Study the drawing (mm; zero at the part's minimum x, y, z) and answer. Coordinates: 2 decimals unless noted, no trailing zeros. Order: outer loops, then holes, each group sorted by start corner. A loop starts at its lowest first (then second) coordinate and runs counter-clockwise, first axis right, second up.
1. The part is cut by section C-C, the plane y = 1. Give the vertices of the cut face in (x, z), then the cut area to 3 significant figures.
2. Flat-ended cylindrical pins translate along their axes: pin 1 Ø2 at (x, z) = (9, 9) entering from -Y; pin 2 Ø8 at (y, z) = (7, 7) entering from -X; pin 3 Ø5.5 at (x, z) = (7.5, 6) entering from +Y; pin 4 Ø1 at (x, z) = (3, 10.5) entering from +Y. Find the tip coordinate at first contact, or state that the pin passes through.
3. Find the intervals of material crossed by probe 1 along X at (y, z) = (6.25, 9); probe 2 along Y at (x, z) = (13.5, 2.5), in increasing order.
4. The part is cut by section D-D, the plane z = 11. Give the vertices of the cut face in (x, y).
5. Determine the mould class of the marked faces 1, 2 and 3 for opening direction Z: +Z half, -Z half, draft (parallel to the pull), parting line (faces both ways), or undercut.
6. The part is cut by section B-B, the plane z = 9. Give the vertices of the cut face in (x, y), then the cut area to 4 significant figures.
7. The part is cut by section A-A, the plane x = 9. Give the vertices of the cut face in (y, z).
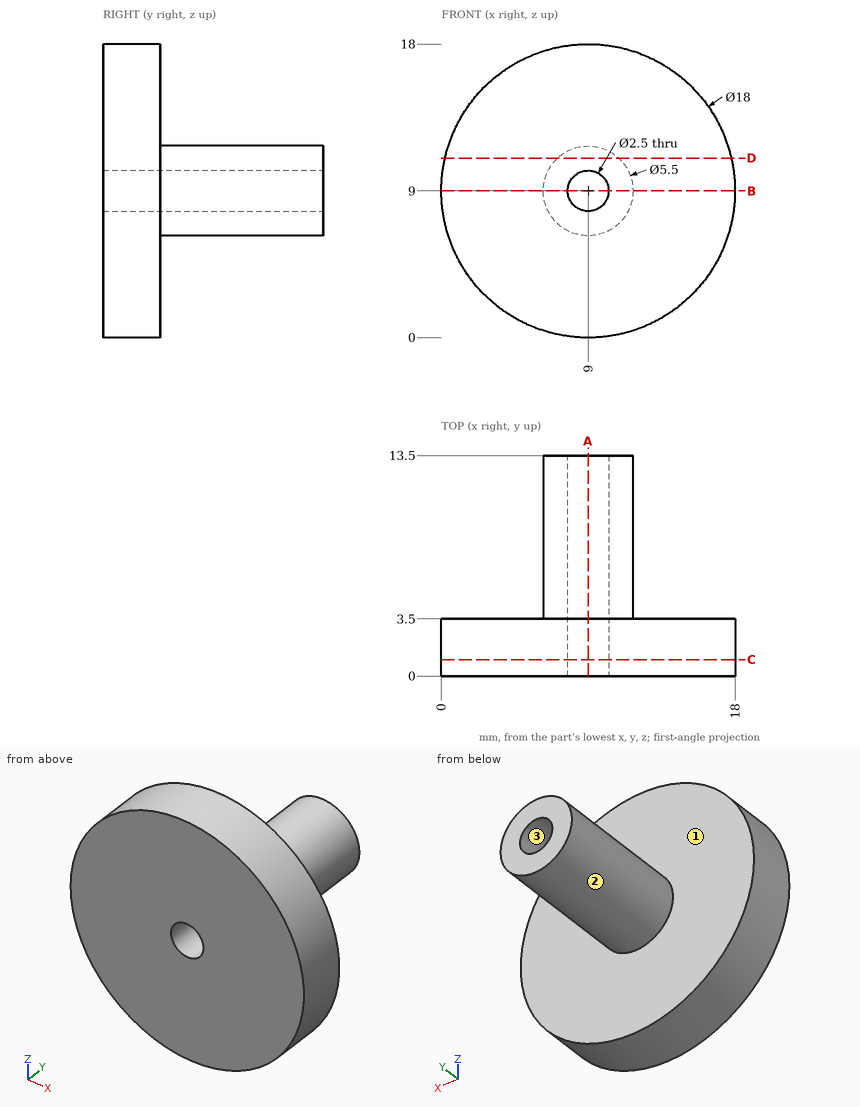
Geometry says:
1. outline: circle Ø18 at (9, 9); hole circle Ø2.5 at (9, 9)
1. area: 250 mm2
2. pin 1: passes through
2. pin 2: stops at x = 0
2. pin 3: stops at y = 13.5
2. pin 4: stops at y = 3.5
3. probe 1: x = 6.25 to 7.75, 10.25 to 11.75
3. probe 2: y = 0 to 3.5
4. outline: (0.23, 0) - (17.77, 0) - (17.77, 3.5) - (10.89, 3.5) - (10.89, 13.5) - (7.11, 13.5) - (7.11, 3.5) - (0.23, 3.5) - close
5. face 1: draft
5. face 2: parting line
5. face 3: undercut
6. outline: (0, 0) - (7.75, 0) - (7.75, 13.5) - (6.25, 13.5) - (6.25, 3.5) - (0, 3.5) - close; (10.25, 0) - (18, 0) - (18, 3.5) - (11.75, 3.5) - (11.75, 13.5) - (10.25, 13.5) - close
6. area: 84.25 mm2
7. outline: (0, 0) - (3.5, 0) - (3.5, 6.25) - (13.5, 6.25) - (13.5, 7.75) - (0, 7.75) - close; (0, 10.25) - (13.5, 10.25) - (13.5, 11.75) - (3.5, 11.75) - (3.5, 18) - (0, 18) - close
